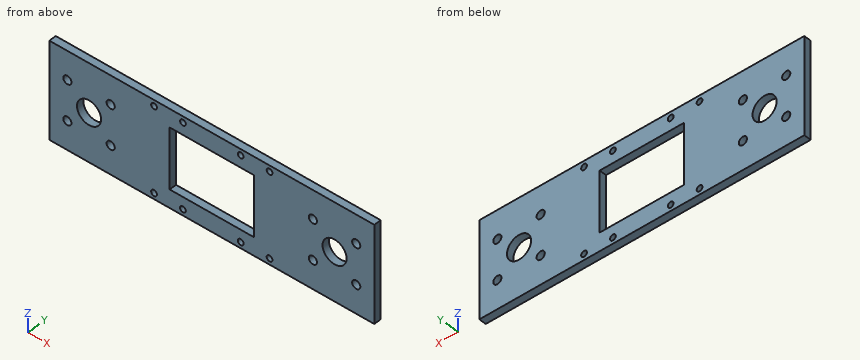
```python
from build123d import *

# Parameters (mm, degrees)
SKETCH1_W           = 135
SKETCH1_H           = 40
SKETCH1_R           = 5
SKETCH1_R_2         = 1.7
SKETCH1_W_2         = 10
SKETCH1_H_2         = 20
BOSS_EXTRUDE1_DEPTH = 3
SKETCH3_R           = 1.2
CUT_EXTRUDE1_DEPTH  = 71.464530084
SKETCH4_W           = 35
SKETCH4_H           = 25
CUT_EXTRUDE2_DEPTH  = 71.464530084


with BuildPart() as part:
    # Sketch1 → Boss-Extrude1 (new body)
    with BuildSketch(Plane(origin=(0, 0, 0), x_dir=(1, 0, 0), z_dir=(0, 1, 0))):
        Rectangle(SKETCH1_W, SKETCH1_H)
        with Locations(Location((-51, 0, 0), (0, 0, 270))):
            Circle(SKETCH1_R, mode=Mode.SUBTRACT)
        with Locations(Location((-60, 8.25, 0), (0, 0, 270))):
            Circle(SKETCH1_R_2, mode=Mode.SUBTRACT)
        with Locations(Location((-42, 8.25, 0), (0, 0, 270))):
            Circle(SKETCH1_R_2, mode=Mode.SUBTRACT)
        with Locations(Location((-42, -8.25, 0), (0, 0, 270))):
            Circle(SKETCH1_R_2, mode=Mode.SUBTRACT)
        with Locations(Location((-60, -8.25, 0), (0, 0, 270))):
            Circle(SKETCH1_R_2, mode=Mode.SUBTRACT)
        with Locations(Location((51, 0, 0), (0, 0, 90))):
            Circle(SKETCH1_R, mode=Mode.SUBTRACT)
        with Locations(Location((42, 8.25, 0), (0, 0, 90))):
            Circle(SKETCH1_R_2, mode=Mode.SUBTRACT)
        with Locations(Location((42, -8.25, 0), (0, 0, 90))):
            Circle(SKETCH1_R_2, mode=Mode.SUBTRACT)
        with Locations(Location((60, -8.25, 0), (0, 0, 90))):
            Circle(SKETCH1_R_2, mode=Mode.SUBTRACT)
        with Locations(Location((60, 8.25, 0), (0, 0, 90))):
            Circle(SKETCH1_R_2, mode=Mode.SUBTRACT)
        Rectangle(SKETCH1_W_2, SKETCH1_H_2, mode=Mode.SUBTRACT)
    extrude(amount=BOSS_EXTRUDE1_DEPTH)

    # Sketch3 → Cut-Extrude1 (cut, through all)
    with BuildSketch(Plane(origin=(0, 3, 0), x_dir=(1, 0, 0), z_dir=(0, 1, 0))):
        with Locations(Location((-12, 17.5, 0), (0, 0, 270))):
            Circle(SKETCH3_R)
        with Locations(Location((-12, -17.5, 0), (0, 0, 90))):
            Circle(SKETCH3_R)
        with Locations(Location((-24, 17.5, 0), (0, 0, 270))):
            Circle(SKETCH3_R)
        with Locations(Location((-24, -17.5, 0), (0, 0, 90))):
            Circle(SKETCH3_R)
        with Locations(Location((24, -17.5, 0), (0, 0, 270))):
            Circle(SKETCH3_R)
        with Locations(Location((24, 17.5, 0), (0, 0, 90))):
            Circle(SKETCH3_R)
        with Locations(Location((12, -17.5, 0), (0, 0, 270))):
            Circle(SKETCH3_R)
        with Locations(Location((12, 17.5, 0), (0, 0, 90))):
            Circle(SKETCH3_R)
    extrude(amount=-CUT_EXTRUDE1_DEPTH, mode=Mode.SUBTRACT)

    # Sketch4 → Cut-Extrude2 (cut, through all)
    with BuildSketch(Plane(origin=(0, 3, 0), x_dir=(1, 0, 0), z_dir=(0, 1, 0))):
        Rectangle(SKETCH4_W, SKETCH4_H)
    extrude(amount=-CUT_EXTRUDE2_DEPTH, mode=Mode.SUBTRACT)


solid = part.part
```
Geometry: final body of the model. Coordinates: model frame, mm. Give positions to 0.01 mm unless a question says otherwise; leave off trailing zeros. Order: outer loops, then holes, each group sorted by start corner. A loop starts at its lowest first (then second) coordinate and runs counter-clockwise, first axis right, second up. Notation, with made-up numbers: M 17,-9.75 L 61,-9.75 A4 ccw 61,-5.75 Z; hole C 27,-24.5 d9. An arc over 180 degrees is marked long. Answer as CSV lines item,"result". Start each with the question number.
1) Cut plane D-D (x = 12). Output: boundary loops of the cut face in (y, z), then the cut area to 3 significant figures.
2) First-contact query: P1, Ø1.4, axis at x = -24, z = -17.5, coming from the -Y side. Flat tip, straight axial feed; report the tip coordinate or a pass-through.
3) Line query: line 1 (X direction, y = 0.85, z = 17.5); line 2 (X direction, y = 2.2, z = -8.25); line 3 (X direction, y = 2.55, z = 0.5). Output: solid intervals per line, ascending. Write a range as from..to.
4) Cut plane C-C (z = -17.5). Output: boundary loops of the cut face in (x, y).
5) Cut plane B-B (y = 2.35). State how many separate pieces and enclosed holes the cut face has, then the cut area to 3 significant figures.
6) Cut plane A-A (x = -7). Output: boundary loops of the cut face in (y, z), then the cut area to 3 significant figures.
Findings below:
1,outline,"M 0,-20 L 3,-20 L 3,-18.7 L 0,-18.7 Z; M 0,-16.3 L 3,-16.3 L 3,-12.5 L 0,-12.5 Z; M 0,12.5 L 3,12.5 L 3,16.3 L 0,16.3 Z; M 0,18.7 L 3,18.7 L 3,20 L 0,20 Z"
1,area,"30.6 mm²"
2,P1,"passes through"
3,line 1,"x = -67.5..-25.2, -22.8..-13.2, -10.8..10.8, 13.2..22.8, 25.2..67.5"
3,line 2,"x = -67.5..-61.7, -58.3..-43.7, -40.3..-17.5, 17.5..40.3, 43.7..58.3, 61.7..67.5"
3,line 3,"x = -67.5..-55.97, -46.03..-17.5, 17.5..46.03, 55.97..67.5"
4,outline,"M -67.5,0 L -25.2,0 L -25.2,3 L -67.5,3 Z; M -22.8,0 L -13.2,0 L -13.2,3 L -22.8,3 Z; M -10.8,0 L 10.8,0 L 10.8,3 L -10.8,3 Z; M 13.2,0 L 22.8,0 L 22.8,3 L 13.2,3 Z; M 25.2,0 L 67.5,0 L 67.5,3 L 25.2,3 Z"
5,separate pieces,"1"
5,enclosed holes,"19"
5,area,"4,260 mm²"
6,outline,"M 0,-20 L 3,-20 L 3,-12.5 L 0,-12.5 Z; M 0,12.5 L 3,12.5 L 3,20 L 0,20 Z"
6,area,"45.0 mm²"
